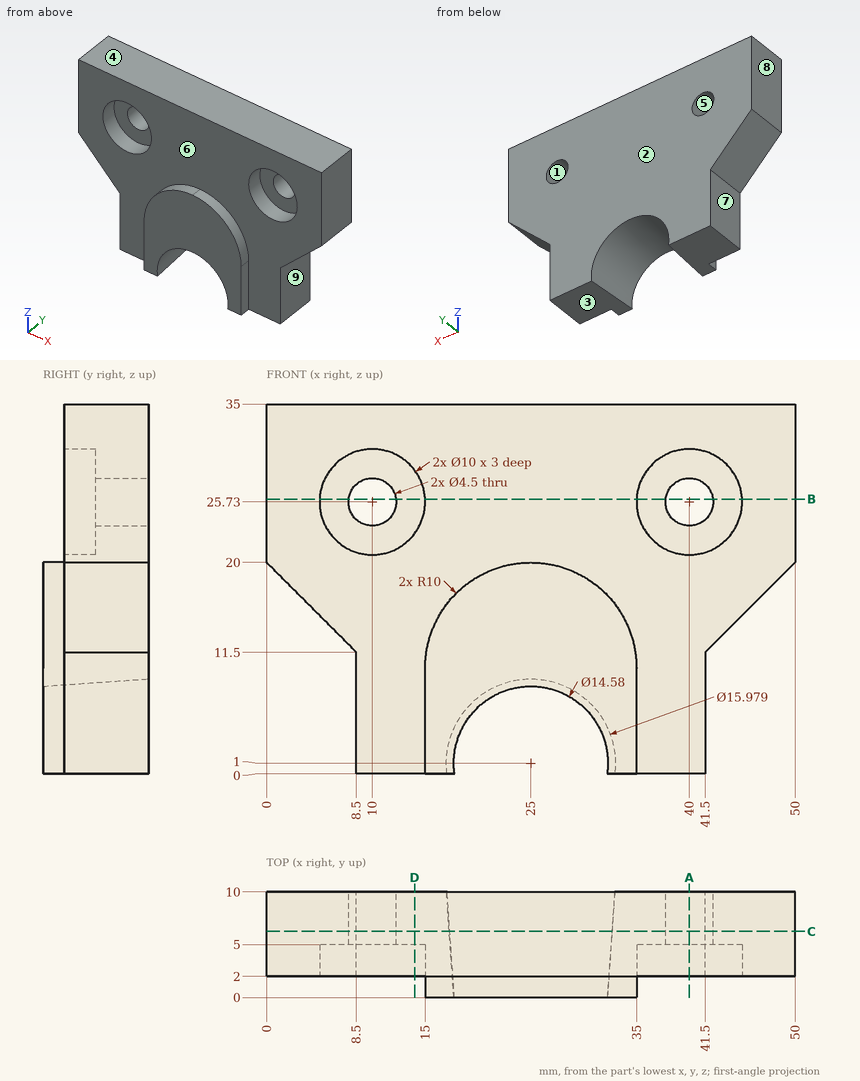
Can you work these out from the drawing? Everything is in mm from the part's minimum corner. A direction names the side the tool comes from. Coordinates: 2 decimals unless noted, no trailing zeros. Loops run counter-clockwise (first coordinate to the right, second up) from the corner with the lowest first, then second, coordinate; pieces in that order, holes last.
1. Imagine slicing it at B-B, the plane z = 26. Please give me the cut outline in (x, y).
2. Imagine slicing it at D-D, the plane x = 14. Please give me the cut outline in (y, z).
3. Imagine slicing it at A-A, the plane x = 40. Please give me the cut outline in (y, z).
4. For the marked faces 5, 6, 7, 8 and 9, which set-ups out of +Z, -Z, +X, -X, +Y, -Y let a thin tool reach every point of the face, with its end or its side?
5. If we mould it in two halves opening along Z, with no side actions, what happens to the marked faces 1, 2, 3 and 4? For each: pulls with the +Z half, pulls with the -Z half, needs draft (parallel to the pull), parting line crosses it, or undercut.
6. I need wall thicknesses on L1, parallel to X at y = 2.25, z = 29.5 (1 decimal); L2, parallel to Y at x = 16.5, z = 20; L3, parallel to Z at x = 39.5, y = 2.75 (1 decimal). Which ranges of each line are inside material? Lowest first, please.
7. Imagine slicing it at C-C, the plane y = 6.25. Count the separate pieces of the cut face and the enclosed holes in it, and give its area (3 significant figures).
8. For P1, Ø1, axis at y = 0.5, z = 2.5, coming from the +X side; P2, Ø6, axis at y = 3.5, z = 14.5, coming from the -X side; P3, Ø13, axis at x = 10, z = 25.73, coming from the -Y side, each with a flat end and sliding along its axis, tell me the tip position at first contact or that it passes through.
Taken from the geometry:
1. outline: (0, 2) - (5.01, 2) - (5.01, 5) - (7.77, 5) - (7.77, 10) - (0, 10) - close; (12.23, 5) - (14.99, 5) - (14.99, 2) - (35.01, 2) - (35.01, 5) - (37.77, 5) - (37.77, 10) - (12.23, 10) - close; (42.23, 5) - (44.99, 5) - (44.99, 2) - (50, 2) - (50, 10) - (42.23, 10) - close
2. outline: (2, 0) - (10, 0) - (10, 35) - (2, 35) - (2, 28.73) - (5, 28.73) - (5, 22.73) - (2, 22.73) - close
3. outline: (2, 0) - (10, 0) - (10, 23.48) - (5, 23.48) - (5, 20.73) - (2, 20.73) - close; (2, 30.73) - (5, 30.73) - (5, 27.98) - (10, 27.98) - (10, 35) - (2, 35) - close
4. face 5: +Y, -Y
4. face 6: +Z, -Y
4. face 7: -Z, -X, +Y, -Y
4. face 8: +Z, -Z, -X, +Y, -Y
4. face 9: -Z, +X, +Y, -Y
5. face 1: undercut
5. face 2: needs draft
5. face 3: pulls with the -Z half
5. face 4: pulls with the +Z half
6. L1: x = 0 to 6.7, 13.3 to 36.7, 43.3 to 50
6. L2: y = 2 to 10
6. L3: z = 0 to 20.8, 30.7 to 35
7. separate pieces: 1
7. enclosed holes: 2
7. area: 1,340 mm2
8. P1: stops at x = 35
8. P2: stops at x = 2.5
8. P3: stops at y = 2
